Source: CAD feature listing. Evaluate the final solid. Frame: model axes, mm. A direction names the side the tool comes from. Round coordinates to 2 decimals unless told otherwise and drop trailing zeros. Order: outer loops, then holes, each group sorted by start corner. A loop starts at its lowest first (then second) coordinate and runs counter-clockwise, first axis right, second up. Notation, with made-up numbers: (53, -10.75) -> (99, -10.75) arc R19 cw to (99, -3.75) -> close; hole circle Ø2 at (80, 13.5). An arc over 180 degrees is marked (long way). Answer as CSV lines item,"result". Start each with the question number.
(1) Section query A-A (x = 0). Output: boundary loops of the cut face in (y, z).
(2) Section query B-B (z = -21). Output: boundary loops of the cut face in (x, y).
(3) Section query D-D (x = -19.5). Output: boundary loops of the cut face in (y, z), plus the area to 3 significant figures.
(4) Line query: line 1 along Z through (x, y) = (0, -1); line 2 along Y through (x, z) = (26, -20); line 3 along X through (y, z) = (1, -34). Output: solid intervals per line, ascending. Write a range as from..to.
(5) Set-up query: faces 4 (the flat face through (-24, 0, -32)), 5 (the flat face through (-22, 22, -29)), 6 (the cylindrical face through (-0.48, 22.18, -70.13)), 7 (the cylindrical face through (0.48, 22.18, 12.36)), 8 (the flat face through (0, -3.11, -28)). Return all of +Z, -Z, +X, -X, +Y, -Y with unobstructed straight access to the full face (end or side cutting, diameter ignored); none if empty.
(6) Pull-direction query (X, two-part tool) for faces 1 (the flat face through (22, 22, -29)), 2 (the flat face through (-32, -2, -29)), 3 (the cylindrical face through (-0.434, -1.533, 19.316)); classes: +X half, -X half, draft (parallel to the pull), parting line (faces both ways), or undercut.
(7) Contact query for flat-ended pins moving along their axis: P1, Ø3, axis at x = 15.5, y = 18, coming from the -Z side; P2, Ø1, axis at x = 10, y = 10, coming from the +Z side; P3, Ø4, axis at y = 36.5, z = 10.5, coming from the -X side. Output: stop coordinate, or through.
(8) Section query C-C (y = 32). Output: boundary loops of the cut face in (x, z).
Autodesk Inventor part; units mm, degrees
ref_plane "YZ Plane" through (0, 0, 0) normal (1, 0, 0) x (0, 1, 0)
ref_plane "XZ Plane" through (0, 0, 0) normal (0, 1, 0) x (-1, 0, 0)
ref_plane "XY Plane" through (0, 0, 0) normal (0, 0, 1) x (1, 0, 0)
sketch "Sketch1" plane through (0, 0, 0) normal (0, 1, 0) x (-1, 0, 0)
  line L0 (0, 12.3635) -> (0, -70.1365) construction
  line L1 (-22, -9.6365) -> (-22, -48.1365)
  line L2 (22, -48.1365) -> (22, -9.6365)
  arc A0 (22, -9.6365) -> (-22, -9.6365) centre (0, -9.6365) ccw
  arc A1 (-22, -48.1365) -> (22, -48.1365) centre (0, -48.1365) ccw
  point P0 (0, 0)
  point P1 (0, -28.8865)
  dimension "d0" = 82.5
  dimension "d1" = 44
extrude "Extrusion1" add sketch "Sketch1" along normal blind 45
sketch "Sketch2" plane through (0, 0, 0) normal (0, -1, 0) x (1, 0, 0)
  arc A0 (22, -9.6365) -> (-22, -9.6365) centre (0, -9.6365) ccw
  line L0 (0, 12.3635) -> (0, -70.1365)
  arc A1 (-22, -48.1365) -> (22, -48.1365) centre (0, -48.1365) ccw
  line L1 (0, -28.8865) -> (22, -28.8865) construction
  line L2 (0, 22.3635) -> (0, -80.1365) construction
  line L3 (-32, -9.6365) -> (-32, -48.1365)
  line L4 (32, -48.1365) -> (32, -9.6365)
  arc A2 (32, -9.6365) -> (-32, -9.6365) centre (0, -9.6365) ccw
  arc A3 (-32, -48.1365) -> (32, -48.1365) centre (0, -48.1365) ccw
  line L5 (22, -9.6365) -> (22, -48.1365)
  line L6 (-22, -48.1365) -> (-22, -9.6365)
  point P0 (0, 0)
  point P1 (8.1717, -6.5277)
  point P2 (0, -80.1365)
  point P3 (0, 22.3635)
  point P4 (0, -70.1365)
  dimension "d8" = 10
  dimension "d9" = 10
  dimension "d10" = 10
extrude "Extrusion2" add sketch "Sketch2" along normal blind 3.11 contours L5 A1 L0 A0 | L0 A1 L6 A0 | A2 L4 A3 L3
sketch "Sketch3" plane through (0, 0, 0) normal (0, 1, 0) x (1, 0, 0)
  circle A0 centre (0, -17.3635) radius 2
  arc A1 (-22, 9.6365) -> (22, 9.6365) centre (0, 9.6365) ccw
  line L0 (-32, 9.6365) -> (-32, 48.1365)
  line L1 (-32, 28.8865) -> (32, 28.8865) construction
  line L2 (32, 48.1365) -> (32, 9.6365)
  circle A2 centre (0, 75.1365) radius 2
  point P0 (0, 0)
  point P1 (0, -12.3635)
  dimension "d13" = 4
  dimension "d14" = 5
extrude "Extrusion3" cut sketch "Sketch3" against normal blind 7.7
properties part number "FabLabPlugwithbottom"
Answer block:
1,outline,"(-3.11, -80.14) -> (0, -80.14) -> (0, -77.14) -> (-3.11, -77.14) -> close; (-3.11, -73.14) -> (0, -73.14) -> (0, -70.14) -> (45, -70.14) -> (45, 12.36) -> (0, 12.36) -> (0, 15.36) -> (-3.11, 15.36) -> close; (-3.11, 19.36) -> (0, 19.36) -> (0, 22.36) -> (-3.11, 22.36) -> close"
2,outline,"(-32, -3.11) -> (32, -3.11) -> (32, 0) -> (22, 0) -> (22, 45) -> (-22, 45) -> (-22, 0) -> (-32, 0) -> close"
3,outline,"(-3.11, -73.51) -> (0, -73.51) -> (0, -58.32) -> (45, -58.32) -> (45, 0.55) -> (0, 0.55) -> (0, 15.74) -> (-3.11, 15.74) -> close"
3,area,"2,930 mm2"
4,line 1,"-80.14..-77.14, -73.14..15.36, 19.36..22.36"
4,line 2,"-3.11..0"
4,line 3,"-22..22"
5,face 4,"+Y"
5,face 5,"+Z, -Z, -X, +Y"
5,face 6,"-Z, +Y"
5,face 7,"+Z, +Y"
5,face 8,"+Z, -Z, +X, -X, -Y"
6,face 1,"+X half"
6,face 2,"-X half"
6,face 3,"undercut"
7,P1,"z = -65.11"
7,P2,"z = 10.21"
7,P3,"x = -12.45"
8,outline,"(-22, -48.14) arc R22 ccw to (22, -48.14) -> (22, -9.64) arc R22 ccw to (-22, -9.64) -> close"
